Autodesk Inventor part; units mm, degrees
ref_plane "YZ Plane" through (0, 0, 0) normal (1, 0, 0) x (0, 1, 0)
ref_plane "XZ Plane" through (0, 0, 0) normal (0, 1, 0) x (-1, 0, 0)
ref_plane "XY Plane" through (0, 0, 0) normal (0, 0, 1) x (1, 0, 0)
sketch "Boceto1" plane through (0, 0, 0) normal (0, 1, 0) x (-1, 0, 0)
  line L0 (18.3875, 12.2875) -> (26.3875, 12.2875)
  line L1 (26.3875, -12.2875) -> (18.3875, -12.2875) construction
  line L2 (26.3875, 18.3875) -> (26.3875, 14.3875)
  line L3 (26.3875, 14.3875) -> (18.3875, 14.3875)
  line L4 (18.3875, 14.3875) -> (18.3875, 12.2875)
  line L5 (18.3875, -12.2875) -> (18.3875, -14.3875) construction
  line L6 (18.3875, -14.3875) -> (26.3875, -14.3875) construction
  line L7 (26.3875, -14.3875) -> (26.3875, -18.3875) construction
  line L8 (18.3875, 18.3875) -> (21.6375, 18.3875)
  line L9 (21.6375, 18.3875) -> (21.6375, 16.8875)
  line L10 (21.6375, 16.8875) -> (23.1375, 16.8875)
  line L11 (23.1375, 16.8875) -> (23.1375, 18.3875)
  line L12 (23.1375, 18.3875) -> (26.3875, 18.3875)
  line L13 (18.3875, -18.3875) -> (21.6375, -18.3875) construction
  line L14 (21.6375, -18.3875) -> (21.6375, -16.8875) construction
  line L15 (21.6375, -16.8875) -> (23.1375, -16.8875) construction
  line L16 (23.1375, -16.8875) -> (23.1375, -18.3875) construction
  line L17 (23.1375, -18.3875) -> (26.3875, -18.3875) construction
  line L18 (0, 0) -> (26.3875, 0)
  line L19 (26.3875, 12.2875) -> (26.3875, 0)
  line L20 (26.3875, 0) -> (26.3875, -12.2875) construction
  arc A0 (18.3875, 18.3875) -> (0, 0) centre (18.3875, 0) ccw
  arc A1 (0, 0) -> (18.3875, -18.3875) centre (18.3875, 0) ccw construction
  point P0 (26.3875, 16.3875)
  point P1 (26.3875, -16.3875)
  dimension "d0" = 24.575
  dimension "d3" = 2.1
  dimension "d4" = 4
  dimension "d5" = 8
  dimension "d6" = 1.5
  dimension "d8" = 3.25
revolve "Revolución1" add sketch "Boceto1" angle 360 about axis through (0, 0, 0) along (-1, 0, 0)
equation "\"d0\" = diametro_agujero_brazo"
equation "\"d3\" = 1.05 * grosor_pared_agujero_brazo"
equation "\"d5\" = profundidad_agujero_brazo"
equation "\"d8\" = -0.5 * d6 + 0.5 * d5"
properties part number "Pata - Pie"
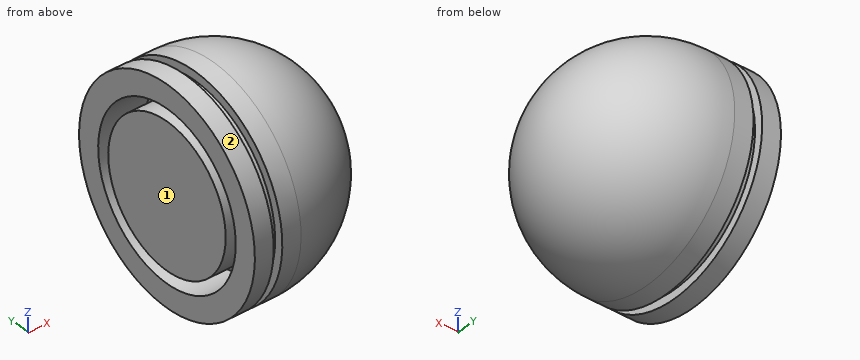
For this review, take the finished solid that the model builds, in its own axes (mm). Face numbers are marked on the shaded views. Coordinates: 2 decimals unless noted, no trailing zeros. Order: outer loops, then holes, each group sorted by start corner. A loop starts at its lowest first (then second) coordinate and runs counter-clockwise, first axis right, second up. Notation, with made-up numbers: (57, -15.75) - (99, -15.75) arc R23 cw to (99, 19.25) - close; hole circle Ø8 at (39, -39.75). An arc over 180 degrees is marked (long way). Answer as CSV lines item,"result". Start each with the question number.
1) To check wall thickness, follow line 1 along Y through (x, z) = (-23.5, 0); line 2 along Y through (x, z) = (-22.25, 0); line 3 along Z through (x, y) = (-21, -7). State the ranges of each line that lie inside material, in increasing order. Write a range as [from, to].
2) Add section B-B (z = 0). State the section outline as (x, y) points (1 decimal).
3) Insertion check: P1, Ø8, axis at x = -16.5, z = -10.5, coming from the +Y side; P2, Ø6, axis at x = -21.5, y = 8.5, coming from the -Z side; P3, Ø1, axis at x = -11, y = -3.5, coming from the -Z side. Each pin has a flat end and moves straight along its axis. Give the tip position at first contact, or say it passes through.
4) Add section D-D (x = -7). State the section outline as (y, z) points.
5) Draft analysis for pull direction Y (two halves, no side actions). For the marked faces 1 and 2, state which applies: +Y half, -Y half, draft (parallel to the pull), parting line (faces both ways), or undercut.
6) Add section A-A (x = -19). State the section outline as (y, z) points (1 decimal).
Result:
1,line 1,"[-18.39, -14.39], [-12.29, 12.29], [14.39, 18.39]"
1,line 2,"[-16.89, -14.39], [-12.29, 12.29], [14.39, 16.89]"
1,line 3,"[-17, -12.57], [-10.1, 10.1], [12.57, 17]"
2,outline,"(-26.4, -18.4) - (-23.1, -18.4) - (-23.1, -16.9) - (-21.6, -16.9) - (-21.6, -18.4) - (-18.4, -18.4) arc R18.4 ccw to (-18.4, 18.4) - (-21.6, 18.4) - (-21.6, 16.9) - (-23.1, 16.9) - (-23.1, 18.4) - (-26.4, 18.4) - (-26.4, 14.4) - (-18.4, 14.4) - (-18.4, 12.3) - (-26.4, 12.3) - (-26.4, -12.3) - (-18.4, -12.3) - (-18.4, -14.4) - (-26.4, -14.4) - close"
3,P1,"y = 17.14"
3,P2,"z = -17.55"
3,P3,"z = -16.71"
4,outline,"circle Ø28.87 at (0, 0)"
5,face 1,"draft"
5,face 2,"parting line"
6,outline,"circle Ø36.8 at (0, 0); circle Ø24.6 at (0, 0); hole circle Ø28.8 at (0, 0)"
